The model under review builds one solid part; all positions refer to its coordinate system, in mm. Coordinates: 2 decimals unless noted, no trailing zeros. Order: outer loops, then holes, each group sorted by start corner. A loop starts at its lowest first (then second) coordinate and runs counter-clockwise, first axis right, second up. Notation, with made-up numbers: M 33.25,46.5 L 84.25,46.5 A16 ccw 84.25,55.5 Z; hole C 61,-22.75 d8. An arc over 180 degrees is marked long. Answer as CSV lines item,"result". Start each with the question number.
Q1. Consider section B-B on y = -228.6. Write out the cut boundary in (x, z) (3 decimals), and give its area (3 significant figures).
Q2. Consider section A-A on x = 0. Write out the cut boundary in (y, z) (3 decimals).
Q3. Consider section C-C on z = -4.5. Write out the cut boundary in (x, y) (3 decimals), and give its area (3 significant figures).
Q4. For P1, Ø4, axis at x = -73, z = -0.5, coming from the +Y side, flat-tipped, find the tip position at first contact; note if it passes through.
Q5. Wall thickness on L1, parallel to Y at x = 0, z = -1.5; L2, parallel to X at y = -224.5, z = 8 (3 decimals); L3, parallel to Y at x = -65, z = -7.75: over which ranges is each line inside the solid? List them lowest first. Write a range as [from, to].
from build123d import *

# Parameters (mm, degrees)
F0_W     = 590.55
F0_H     = 19.05
F1_DEPTH = 1200.15
F3_D     = 152.4


with BuildPart() as f1:
    # F0 (on Front) → F1 (new body)
    with BuildSketch(Plane.XZ):
        Rectangle(F0_W, F0_H)
    extrude(amount=F1_DEPTH)

    # F3 (through all)
    with Locations(Plane.XY.offset(9.525)):
        with Locations((0, -228.6)):
            Hole(F3_D / 2)


solid = f1.part
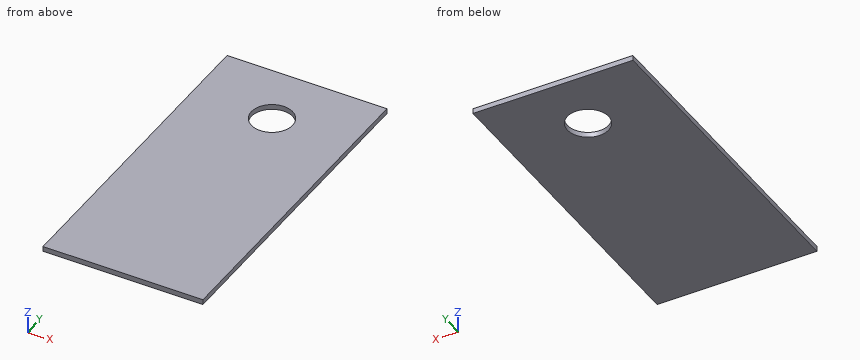
Evaluation:
1,outline,"M -295.275,-9.525 L -76.2,-9.525 L -76.2,9.525 L -295.275,9.525 Z; M 76.2,-9.525 L 295.275,-9.525 L 295.275,9.525 L 76.2,9.525 Z"
1,area,"8,350 mm²"
2,outline,"M -1200.15,-9.525 L -304.8,-9.525 L -304.8,9.525 L -1200.15,9.525 Z; M -152.4,-9.525 L 0,-9.525 L 0,9.525 L -152.4,9.525 Z"
3,outline,"M -295.275,-1200.15 L 295.275,-1200.15 L 295.275,0 L -295.275,0 Z; hole C 0,-228.6 d152.4"
3,area,"691,000 mm²"
4,P1,"stops at y = 0"
5,L1,"y = [-1200.15, -304.8], [-152.4, 0]"
5,L2,"x = [-295.275, -76.09], [76.09, 295.275]"
5,L3,"y = [-1200.15, -268.37], [-188.83, 0]"
